from build123d import *

# Parameters (mm, degrees)
F0_R     = 0.5
F0_R_2   = 1.13
F1_DEPTH = 1.61
F0_W     = 7.5
F0_H     = 4.64
F0_H_2   = 1.06
F2_DEPTH = 4.11


with BuildPart() as f1:
    # F0 (on Top) → F1 (new body)
    with BuildSketch(Plane.XY):
        Polygon((-10.25, -5.75), (10.25, -5.75), (10.25, 5.75), (3.75, 5.75), (3.75, 1.11), (-3.75, 1.11), (-3.75, 5.75), (-10.25, 5.75), align=None)
        with Locations((-5.08, -4.1)):
            Circle(F0_R, mode=Mode.SUBTRACT)
        with Locations((-2.54, -4.1)):
            Circle(F0_R, mode=Mode.SUBTRACT)
        with Locations((0, -4.1)):
            Circle(F0_R, mode=Mode.SUBTRACT)
        with Locations((2.54, -4.1)):
            Circle(F0_R, mode=Mode.SUBTRACT)
        with Locations((5.08, -4.1)):
            Circle(F0_R, mode=Mode.SUBTRACT)
        with Locations((-7.77, 3.27)):
            Circle(F0_R_2, mode=Mode.SUBTRACT)
        with Locations((7.77, 3.27)):
            Circle(F0_R_2, mode=Mode.SUBTRACT)
    extrude(amount=F1_DEPTH)

    # F0 (on Top) → F2 (join)
    with BuildSketch(Plane.XY):
        with Locations((0, 3.43)):
            Rectangle(F0_W, F0_H)
        with Locations((0, 6.28)):
            Rectangle(F0_W, F0_H_2)
    extrude(amount=F2_DEPTH)


solid = f1.part
Here's how the part is built. I have some questions about the finished solid (model axes, mm). A direction names the side the tool comes from. Give positions to 0.01 mm unless a question says otherwise; leave off trailing zeros. Order: outer loops, then holes, each group sorted by start corner. A loop starts at its lowest first (then second) coordinate and runs counter-clockwise, first axis right, second up. Notation, with made-up numbers: M 37.5,73 L 84.5,73 A17 cw 84.5,94 Z; hole C -15.5,68.5 d2. An arc over 180 degrees is marked long. Answer as a JSON object with one key per item and string values. Group by question number.
1) Suppose I cut it at D-D, the plane y = -4.1. Write out the boundary of the cut face in (x, z), plus the area to 3 significant figures.
2) Suppose I cut it at A-A, the plane x = 5.08. Write out the boundary of the cut face in (y, z).
3) Please list where these lines run through material, in increasing order: L1, parallel to Y at x = 7.77, z = 0.45; L2, parallel to Y at x = -2.5, z = 1.05; L3, parallel to X at y = 2.5, z = 0.55. Write a range as [from, to].
4) Suppose I cut it at B-B, the plane z = 1. Write out the boundary of the cut face in (x, y), plus the area to 3 significant figures.
5) I'm going to push flat-ended pins straight in: pin 1 Ø0.8 at (x, z) = (1.5, 2.5) entering from -Y; pin 2 Ø1.2 at (y, z) = (3, 2.5) entering from -X; pin 3 Ø2 at (x, y) = (-5.5, 2) entering from +Z. Where does each tip first touch, or does it pass through?
6) Suppose I cut it at C-C, the plane y = 3.27. Write out the boundary of the cut face in (x, z), plus the area to 3 significant figures.
7) We'd pull the mould along Y, two halves only. Please class faces 1 (the cylindrical face through (-8.603, 4.034, 0.794)), 2 (the flat face through (0, -5.75, 1)), 3 (the flat face through (-3.75, 5, 2)), 4 (the cylindrical face through (3, -3.9, 0.8)): pulls with the +Y half, pulls with the -Y half, needs draft (parallel to the pull), parting line crosses it, or undercut.
8) On a 3-axis mill with a long thin cutter (end or side, diameter ignored), from which of +Z, -Z, +X, -X, +Y, -Y can I reach the whole of each face in a straight line? I mean faces 5 (the flat face through (7, 5.75, 1)), 6 (the cylindrical face through (4.68, -4.4, 0.79)), 7 (the flat face through (0, 0, 1.61)), 8 (the flat face through (0, 1.11, 3)), 9 (the flat face through (-7, 5.75, 1)). Say none if no direction works.
Results found:
{
 "1": {"outline": "M -10.25,0 L -5.58,0 L -5.58,1.61 L -10.25,1.61 Z; M -4.58,0 L -3.04,0 L -3.04,1.61 L -4.58,1.61 Z; M -2.04,0 L -0.5,0 L -0.5,1.61 L -2.04,1.61 Z; M 0.5,0 L 2.04,0 L 2.04,1.61 L 0.5,1.61 Z; M 3.04,0 L 4.58,0 L 4.58,1.61 L 3.04,1.61 Z; M 5.58,0 L 10.25,0 L 10.25,1.61 L 5.58,1.61 Z", "area": "25.0 mm²"},
 "2": {"outline": "M -5.75,0 L -4.6,0 L -4.6,1.61 L -5.75,1.61 Z; M -3.6,0 L 5.75,0 L 5.75,1.61 L -3.6,1.61 Z"},
 "3": {"L1": "[-5.75, 2.14], [4.4, 5.75]", "L2": "[-5.75, -4.6], [-3.6, 6.81]", "L3": "[-10.25, -8.6], [-6.94, 6.94], [8.6, 10.25]"},
 "4": {"outline": "M -10.25,-5.75 L 10.25,-5.75 L 10.25,5.75 L 3.75,5.75 L 3.75,6.81 L -3.75,6.81 L -3.75,5.75 L -10.25,5.75 Z; hole C -7.77,3.27 d2.26; hole C -5.08,-4.1 d1; hole C -2.54,-4.1 d1; hole C 0,-4.1 d1; hole C 2.54,-4.1 d1; hole C 5.08,-4.1 d1; hole C 7.77,3.27 d2.26", "area": "232 mm²"},
 "5": {"pin 1": "y = 1.11", "pin 2": "x = -3.75", "pin 3": "z = 1.61"},
 "6": {"outline": "M -10.25,0 L -8.9,0 L -8.9,1.61 L -10.25,1.61 Z; M -6.64,0 L 6.64,0 L 6.64,1.61 L 3.75,1.61 L 3.75,4.11 L -3.75,4.11 L -3.75,1.61 L -6.64,1.61 Z; M 8.9,0 L 10.25,0 L 10.25,1.61 L 8.9,1.61 Z", "area": "44.5 mm²"},
 "7": {"face 1": "undercut", "face 2": "pulls with the -Y half", "face 3": "needs draft", "face 4": "undercut"},
 "8": {"face 5": "+Z, -Z, +X, +Y", "face 6": "+Z, -Z", "face 7": "+Z, -Y", "face 8": "+Z, +X, -X, -Y", "face 9": "+Z, -Z, -X, +Y"}
}
